Autodesk Inventor part; units mm, degrees
ref_plane "YZ Plane" through (0, 0, 0) normal (1, 0, 0) x (0, 1, 0)
ref_plane "XZ Plane" through (0, 0, 0) normal (0, 1, 0) x (-1, 0, 0)
ref_plane "XY Plane" through (0, 0, 0) normal (0, 0, 1) x (1, 0, 0)
sketch "Sketch1" plane through (0, 0, 0) normal (0, 1, 0) x (-1, 0, 0)
  circle A0 centre (0, 0) radius 17.399
  circle A1 centre (0, -38.1) radius 17.399
  circle A2 centre (0, -76.2) radius 17.399
  line L0 (20.65, 20.65) -> (-20.65, 20.65)
  line L1 (-20.65, 20.65) -> (-20.65, -96.85)
  line L2 (-20.65, -96.85) -> (20.65, -96.85)
  line L3 (20.65, -96.85) -> (20.65, 20.65)
  dimension "d0" = 34.798
  dimension "d1" = 34.798
  dimension "d2" = 38.1
  dimension "d3" = 34.798
  dimension "d4" = 38.1
  dimension "d5" = 20.65
  dimension "d6" = 20.65
  dimension "d7" = 20.65
  dimension "d8" = 20.65
extrude "Extrusion1" add sketch "Sketch1" along normal blind 25
extrude "Extrusion2" add sketch "Sketch1" along normal blind 6.35 contours A0 | A1 | A2
fillet "Fillet1" radius 3.175 8 edges at (20.65, 12.5, 20.65) (-20.65, 12.5, 20.65) (20.65, 12.5, -96.85) (-20.65, 12.5, -96.85) (0, 25, -96.85) (0, 25, 20.65) (20.65, 25, -38.1) (-20.65, 25, -38.1)
sketch "Sketch3" plane through (-20.65, 0, -93.675) normal (-1, 0, 0) x (0, 0, 1)
  circle A0 centre (55.5752, 10.9157) radius 5
  line L0 (0, 0) -> (0, 21.825)
  line L1 (0, 21.825) -> (111.15, 21.825)
  point P0 (93.675, 0)
  dimension "d19" = 10
  dimension "d20" = 55.5752
  dimension "d21" = 10.9093
extrude "Extrusion4" cut sketch "Sketch3" against normal blind 3
sketch "Sketch4" plane through (-17.475, 0, 20.65) normal (0, 0, 1) x (1, 0, 0)
  circle A0 centre (17.4752, 10.9157) radius 5
  line L0 (0, 0) -> (0, 21.825)
  line L1 (0, 21.825) -> (34.95, 21.825)
  point P0 (17.475, 0)
  dimension "d24" = 10
  dimension "d25" = 17.4752
  dimension "d26" = 10.9093
extrude "Extrusion5" cut sketch "Sketch4" against normal blind 3
sketch "Sketch5" plane through (20.65, 0, 17.475) normal (1, 0, 0) x (0, 0, -1)
  circle A0 centre (55.5748, 10.9157) radius 5
  circle A1 centre (55.5748, 10.9157) radius 5
  point P0 (17.475, 0)
  dimension "d29" = 10
extrude "Extrusion6" cut sketch "Sketch5" against normal blind 3
sketch "Sketch6" plane through (17.475, 0, -96.85) normal (0, 0, -1) x (-1, 0, 0)
  circle A0 centre (17.4748, 10.9157) radius 5
  circle A1 centre (17.4748, 10.9157) radius 5
  point P0 (17.475, 0)
extrude "Extrusion7" cut sketch "Sketch6" against normal blind 3
properties part number "_3DPrint"
Source: CAD feature listing. Evaluate the final solid. Frame: model axes, mm. A direction names the side the tool comes from. Coordinates: 2 decimals unless noted, no trailing zeros. Order: outer loops, then holes, each group sorted by start corner. A loop starts at its lowest first (then second) coordinate and runs counter-clockwise, first axis right, second up. Notation, with made-up numbers: M 33.25,-2.5 L 40.25,-2.5 A9 cw 40.25,4.5 Z; hole C 71.5,25 d4. An arc over 180 degrees is marked long. Write each question's results on one line, items separated by ' | '. Start each with the question number.
1) Line query: line 1 (Z direction, x = 0, y = 14); line 2 (Z direction, x = 7, y = 12); line 3 (Y direction, x = 2, z = -37.5). Output: solid intervals per line, ascending. Write a range as from..to.
2) Access query for faces 4 (the face through (3.968, 7.873, -95.371)), 5 (the face through (-3.968, 7.873, 19.171)), 6 (the face through (19.74, 11.07, -95.9)), 7 (the face through (0, 6.35, 0)), 8 (the face through (-19.171, 11.136, -43.095)). Directions: +Z, -Z, +X, -X, +Y, -Y. A direction counts if a zero-diameter tool reaches every point of the face in a straight line with its end or side. Return the directions, or none.
3) Draft query along Y for faces 1 (the face through (13, 25, -50)), 2 (the face through (3.772, 15.544, -21.115)), 3 (the face through (0, 11, -93.85)). Return one class per face: released by +Y, released by -Y, zero draft, split by the parting line, or undercut.
4) Section query B-B (x = 0). Return the cut outline in (y, z) (3 decimals).
5) Section query D-D (x = -14). Return the cut outline in (y, z) (3 decimals).
6) Section query C-C (z = -76.2). Return the cut outline in (x, y) (3 decimals).
7) Section query A-A (z = -38.1). Return the cut outline in (x, y) (3 decimals), plus the area to 3 significant figures.
8) Contact query for flat-ended pins moving along their axis: pin 1 Ø4 at (x, y) = (-0.5, 12.5) entering from +Z; pin 2 Ø3 at (y, z) = (11, -37.5) entering from +X; pin 3 Ø10.5 at (x, z) = (0, -78.5) entering from +Y; pin 4 Ø21 at (x, z) = (0, -38.1) entering from -Y. Output: stop coordinate, or through.
Answers:
1) line 1: z = -93.85..-93.6, -58.8..-55.5, -20.7..-17.4, 17.4..17.65 | line 2: z = -96.85..-92.13, -60.27..-54.03, -22.17..-15.93, 15.93..20.65 | line 3: y = 0..6.35
2) face 4: -Z | face 5: +Z | face 6: -Z, +X, +Y, -Y | face 7: +Y | face 8: -X
3) face 1: released by +Y | face 2: zero draft | face 3: undercut
4) outline: M 0,-96.85 L 5.916,-96.85 L 5.916,-93.85 L 15.916,-93.85 L 15.916,-96.85 L 21.825,-96.85 A3.175 ccw 25,-93.675 L 25,-93.599 L 6.35,-93.599 L 6.35,-58.801 L 25,-58.801 L 25,-55.499 L 6.35,-55.499 L 6.35,-20.701 L 25,-20.701 L 25,-17.399 L 6.35,-17.399 L 6.35,17.399 L 25,17.399 L 25,17.475 A3.175 ccw 21.825,20.65 L 15.916,20.65 L 15.916,17.65 L 5.916,17.65 L 5.916,20.65 L 0,20.65 Z
5) outline: M 0,-96.85 L 21.825,-96.85 A3.175 ccw 25,-93.675 L 25,-86.531 L 6.35,-86.531 L 6.35,-65.869 L 25,-65.869 L 25,-48.431 L 6.35,-48.431 L 6.35,-27.769 L 25,-27.769 L 25,-10.331 L 6.35,-10.331 L 6.35,10.331 L 25,10.331 L 25,17.475 A3.175 ccw 21.825,20.65 L 0,20.65 Z
6) outline: M -20.65,0 L 20.65,0 L 20.65,21.825 A3.175 ccw 17.475,25 L 17.399,25 L 17.399,6.35 L -17.399,6.35 L -17.399,25 L -17.475,25 A3.175 ccw -20.65,21.825 Z
7) outline: M -20.65,0 L 20.65,0 L 20.65,5.916 L 17.65,5.916 L 17.65,15.916 L 20.65,15.916 L 20.65,21.825 A3.175 ccw 17.475,25 L 17.399,25 L 17.399,6.35 L -17.399,6.35 L -17.399,25 L -17.475,25 A3.175 ccw -20.65,21.825 L -20.65,15.916 L -17.65,15.916 L -17.65,5.916 L -20.65,5.916 Z | area: 319 mm^2
8) pin 1: stops at z = 17.65 | pin 2: stops at x = 17.65 | pin 3: stops at y = 6.35 | pin 4: stops at y = 0
